```python
from build123d import *

# Parameters (mm, degrees)
SKETCH1_W           = 44.45
SKETCH1_H           = 158.75
BOSS_EXTRUDE1_DEPTH = 4.7625
CUT_EXTRUDE1_DEPTH  = 5.7625


with BuildPart() as part:
    # Sketch1 → Boss-Extrude1 (new body)
    with BuildSketch(Plane(origin=(0, 0, 0), x_dir=(1, 0, 0), z_dir=(0, 1, 0))):
        Rectangle(SKETCH1_W, SKETCH1_H)
    extrude(amount=BOSS_EXTRUDE1_DEPTH)

    # Sketch2 → Cut-Extrude1 (cut, through all)
    with BuildSketch(Plane(origin=(0, 4.7625, 0), x_dir=(1, 0, 0), z_dir=(0, 1, 0))):
        with BuildLine():
            Line((0, 50.8), (0, 69.85))
            ThreePointArc((0, 69.85), (-3.175, 73.025), (-6.35, 69.85))
            Line((-6.35, 69.85), (-6.35, 50.8))
            ThreePointArc((-6.35, 50.8), (-3.175, 47.625), (0, 50.8))
        make_face()
        with BuildLine():
            Line((-6.35, -50.8), (-6.35, -69.85))
            ThreePointArc((-6.35, -69.85), (-3.175, -73.025), (0, -69.85))
            Line((0, -69.85), (0, -50.8))
            ThreePointArc((0, -50.8), (-3.175, -47.625), (-6.35, -50.8))
        make_face()
    extrude(amount=-CUT_EXTRUDE1_DEPTH, mode=Mode.SUBTRACT)


solid = part.part
```
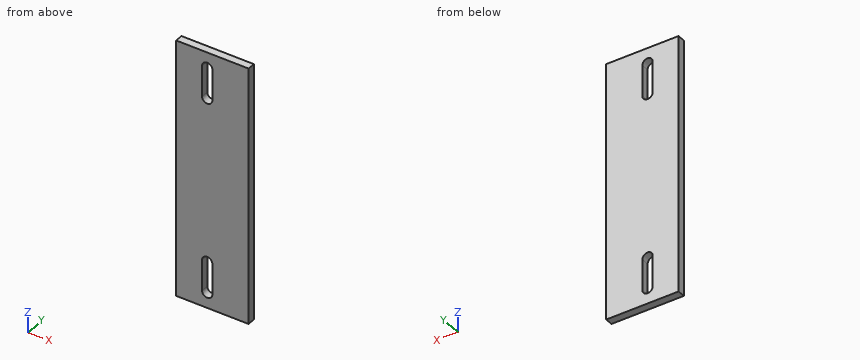
Geometry: final body of the model. Coordinates: model frame, mm. Coordinates: 2 decimals unless noted, no trailing zeros. Order: outer loops, then holes, each group sorted by start corner. A loop starts at its lowest first (then second) coordinate and runs counter-clockwise, first axis right, second up. Notation, with made-up numbers: M 1.5,76.25 L 58.5,76.25 A21 ccw 58.5,103.25 Z; hole C 75,0.5 d1. An arc over 180 degrees is marked long. Answer in a Markdown table with one row per item. Add a question column.
Q1. Section query B-B on y = 2.95. Return the cut outline in (x, z) (3 decimals), and give its area (3 significant figures).
Q2. Section query C-C on x = -4. Return the cut outline in (y, z) (1 decimal).
Q3. Line query: L1, parallel to Z at x = -3, y = 4.15 (3 decimals); L2, parallel to X at y = 3.55, z = 70 (3 decimals); L3, parallel to Z at x = -5.5, y = 2.8 (3 decimals). Output: solid intervals per line, ascending.
Completed:
| question | item | result |
|---|---|---|
| 1 | outline | M -22.225,-79.375 L 22.225,-79.375 L 22.225,79.375 L -22.225,79.375 Z; hole M -6.35,-69.85 A3.175 ccw 0,-69.85 L 0,-50.8 A3.175 ccw -6.35,-50.8 Z; hole M -6.35,50.8 A3.175 ccw 0,50.8 L 0,69.85 A3.175 ccw -6.35,69.85 Z |
| 1 | area | 6,750 mm2 |
| 2 | outline | M 0,-79.4 L 4.8,-79.4 L 4.8,-72.9 L 0,-72.9 Z; M 0,-47.7 L 4.8,-47.7 L 4.8,47.7 L 0,47.7 Z; M 0,72.9 L 4.8,72.9 L 4.8,79.4 L 0,79.4 Z |
| 3 | L1 | z = -79.375 to -73.02, -47.63 to 47.63, 73.02 to 79.375 |
| 3 | L2 | x = -22.225 to -6.346, -0.004 to 22.225 |
| 3 | L3 | z = -79.375 to -72.012, -48.638 to 48.638, 72.012 to 79.375 |
